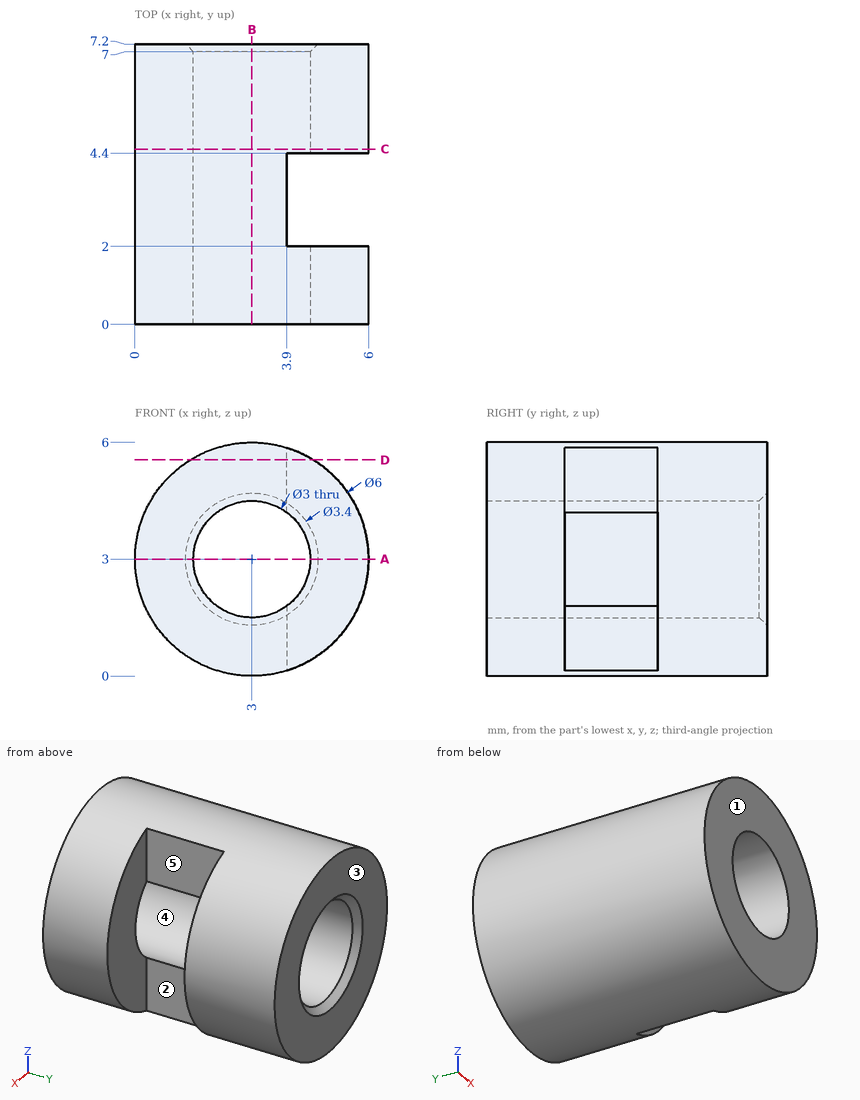
Input: dimensioned drawing with shaded views. Units: mm. Origin: part minimum x, y, z. A direction names the side the tool comes from. Round coordinates to 2 decimals unless told otherwise and drop trailing zeros. Loops run counter-clockwise (first coordinate to the right, second up) from the corner with the lowest first, then second, coordinate; pieces in that order, holes last. Notation, with made-up numbers: (3, 59) -> (46, 59) arc R17 ccw to (46, 76) -> close; hole circle Ø3 at (36, 3). An arc over 180 degrees is marked (long way). Answer as a JSON object with one key per item and string values. Group by question number.
1) Section query A-A on z = 3. Output: boundary loops of the cut face in (x, y).
2) Reachability of the marked faces 4 and 5 from +Z, -Z, +X, -X, +Y, -Y: full face, straight path, thin tool, end or side. Return the list, or none.
3) Section query B-B on x = 3. Output: boundary loops of the cut face in (y, z).
4) Draft query along Y for the marked faces 1, 2 and 3. Return one class per face: +Y half, -Y half, draft (parallel to the pull), parting line (faces both ways), or undercut.
5) Ray query, L1, parallel to Y at x = 5.3, z = 2.5; L2, parallel to Z at x = 3, y = 3.25; L3, parallel to X at y = 0.5, z = 3.75. Return the intervals inside material, ascending.
6) Pin query (flat end, axial travel): pin 1 (1.8 mm diameter, centred on y = 3, z = 4.5, fed in from +X); pin 2 (2 mm diameter, centred on x = 1.5, y = 6, fed in from -Z). Return the tip coordinate at first contact, or that it passes through.
7) Section query C-C on y = 4.5. Output: boundary loops of the cut face in (x, z), plus the area to 3 significant figures.
8) Section query D-D on z = 5.55. Output: boundary loops of the cut face in (x, y), plus the area to 3 significant figures.
Reply:
{
 "1": {"outline": "(0, 0) -> (1.5, 0) -> (1.5, 7) -> (1.3, 7.2) -> (0, 7.2) -> close; (4.5, 0) -> (6, 0) -> (6, 2) -> (4.5, 2) -> close; (4.5, 4.4) -> (6, 4.4) -> (6, 7.2) -> (4.7, 7.2) -> (4.5, 7) -> close"},
 "2": {"face 4": "+Y, -Y", "face 5": "+Z, -Z, +X"},
 "3": {"outline": "(0, 0) -> (7.2, 0) -> (7.2, 1.3) -> (7, 1.5) -> (0, 1.5) -> close; (0, 4.5) -> (7, 4.5) -> (7.2, 4.7) -> (7.2, 6) -> (0, 6) -> close"},
 "4": {"face 1": "-Y half", "face 2": "undercut", "face 3": "+Y half"},
 "5": {"L1": "y = 0 to 2, 4.4 to 7.2", "L2": "z = 0 to 1.5, 4.5 to 6", "L3": "x = 0.1 to 1.7, 4.3 to 5.9"},
 "6": {"pin 1": "stops at x = 3.9", "pin 2": "stops at z = 0.04"},
 "7": {"outline": "circle Ø6 at (3, 3); hole circle Ø3 at (3, 3)", "area": "21.2 mm2"},
 "8": {"outline": "(1.42, 0) -> (4.58, 0) -> (4.58, 2) -> (3.9, 2) -> (3.9, 4.4) -> (4.58, 4.4) -> (4.58, 7.2) -> (1.42, 7.2) -> close", "area": "21.1 mm2"}
}
